Check sheet for the modelled part. Datum: model origin and axes. Units: mm. Coordinates: 2 decimals unless noted, no trailing zeros. Loops run counter-clockwise (first coordinate to the right, second up) from the corner with the lowest first, then second, coordinate; pieces in that order, holes last. Notation, with made-up numbers: (-14, -31) - (45, -31) arc R24 ccw to (45, -20) - close; hole circle Ø7 at (54, 57.25). An arc over 180 degrees is marked (long way). Use a Markdown table: item, result. Add a question column.
1) Sectioned sample at A-A, the plane y = 7.5. Enter the section's corners in (x, z).
2) Draft check along X on faces 1 (the flat face through (4, 13, 12.7)), 2 (the flat face through (10.2, 7.7, -10.2)), 3 (the cylindrical face through (-4.42, 11.56, -9.35)). Enter one of: pulls with the +X half, pulls with the -X half, needs draft (parallel to the pull), parting line crosses it, or undercut.
3) Sectioned sample at B-B, the plane z = 0. Enter the section's corners in (x, y), then the cut area to 3 significant figures.
4) Sectioned sample at D-D, the plane y = -1.75. Enter the section's corners in (x, z).
5) Sectioned sample at C-C, the plane x = -8.5. Enter the section's corners in (y, z).
6) Thickness scan on line 1 (Y direction, x = 0, z = -8); line 2 (Z direction, x = 0, y = 18). Record the ranges inside material, lowest first.
7) Go/stop test with flat-tipped pins: P1, Ø2, axis at y = 12.5, z = -9, coming from the +X side; P2, Ø11, axis at x = 0, z = 0, coming from the -Y side; P3, Ø3, axis at y = 3, z = -10, coming from the +X side. Record where each tip stops, or that it passes through.
from build123d import *

# Parameters (mm, degrees)
SKETCH1_R           = 6
BOSS_EXTRUDE1_DEPTH = 15
SKETCH2_R           = 6
CUT_EXTRUDE1_DEPTH  = 32
SKETCH3_R           = 6
CUT_EXTRUDE2_DEPTH  = 32
BOSS_EXTRUDE2_DEPTH = 5
BOSS_EXTRUDE3_DEPTH = 5
CUT_EXTRUDE3_START  = -31
SKETCH8_R           = 6
CUT_EXTRUDE3_DEPTH  = 31


with BuildPart() as part:
    # Sketch1 → Boss-Extrude1 (new body)
    with BuildSketch(Plane(origin=(0, 0, 0), x_dir=(1, 0, 0), z_dir=(0, 1, 0))):
        Polygon((-7.7, 12.7), (-12.7, 7.7), (-12.7, -7.7), (-7.7, -12.7), (7.7, -12.7), (12.7, -7.7), (12.7, 7.7), (7.7, 12.7), align=None)
        with Locations(Location((0, 0, 0), (0, 0, 270))):
            Circle(SKETCH1_R, mode=Mode.SUBTRACT)
    extrude(amount=BOSS_EXTRUDE1_DEPTH)

    # Sketch2 → Cut-Extrude1 (cut)
    with BuildSketch(Plane.XY.offset(12.7)):
        with Locations((0, 7.5)):
            Circle(SKETCH2_R)
    extrude(amount=-CUT_EXTRUDE1_DEPTH, mode=Mode.SUBTRACT)

    # Sketch3 → Cut-Extrude2 (cut)
    with BuildSketch(Plane.ZY.offset(12.7)):
        with Locations((0, 7.5)):
            Circle(SKETCH3_R)
    extrude(amount=-CUT_EXTRUDE2_DEPTH, mode=Mode.SUBTRACT)

    # Sketch6 → Boss-Extrude2 (add)
    with BuildSketch(Plane(origin=(0, 15, 0), x_dir=(1, 0, 0), z_dir=(0, 1, 0))):
        Polygon((7.7, 12.7), (-7.7, 12.7), (-12.7, 7.7), (-12.7, -7.7), (-7.7, -12.7), (7.7, -12.7), (12.7, -7.7), (12.7, 7.7), align=None)
    extrude(amount=BOSS_EXTRUDE2_DEPTH)

    # Sketch7 → Boss-Extrude3 (add)
    with BuildSketch(Plane.XZ):
        Polygon((-7.7, -12.7), (7.7, -12.7), (12.7, -7.7), (12.7, 7.7), (7.7, 12.7), (-7.7, 12.7), (-12.7, 7.7), (-12.7, -7.7), align=None)
    extrude(amount=BOSS_EXTRUDE3_DEPTH)

    # Sketch8 → Cut-Extrude3 (cut)
    with BuildSketch(Plane(origin=(0, 20, 0), x_dir=(1, 0, 0), z_dir=(0, 1, 0)).offset(CUT_EXTRUDE3_START)):
        with Locations(Location((0, 0, 0), (0, 0, 135))):
            Circle(SKETCH8_R)
    extrude(amount=CUT_EXTRUDE3_DEPTH, mode=Mode.SUBTRACT)


solid = part.part
Solved:
| question | item | result |
|---|---|---|
| 1 | outline | (-12.7, -7.7) - (-7.7, -12.7) - (-6, -12.7) - (-6, -6) - (-12.7, -6) - close; (-12.7, 6) - (-6, 6) - (-6, 12.7) - (-7.7, 12.7) - (-12.7, 7.7) - close; (6, -12.7) - (7.7, -12.7) - (12.7, -7.7) - (12.7, -6) - (6, -6) - close; (6, 6) - (12.7, 6) - (12.7, 7.7) - (7.7, 12.7) - (6, 12.7) - close |
| 2 | face 1 | needs draft |
| 2 | face 2 | pulls with the +X half |
| 2 | face 3 | undercut |
| 3 | outline | (-12.7, -5) - (-6, -5) - (-6, 1.5) - (-12.7, 1.5) - close; (-12.7, 13.5) - (-6, 13.5) - (-6, 20) - (-12.7, 20) - close; (6, -5) - (12.7, -5) - (12.7, 1.5) - (6, 1.5) - close; (6, 13.5) - (12.7, 13.5) - (12.7, 20) - (6, 20) - close |
| 3 | area | 174 mm2 |
| 4 | outline | (-12.7, -7.7) - (-7.7, -12.7) - (7.7, -12.7) - (12.7, -7.7) - (12.7, 7.7) - (7.7, 12.7) - (-7.7, 12.7) - (-12.7, 7.7) - close; hole circle Ø12 at (0, 0) |
| 5 | outline | (-5, -11.9) - (20, -11.9) - (20, 11.9) - (-5, 11.9) - close; hole circle Ø12 at (7.5, 0) |
| 6 | line 1 | y = -5 to 1.5, 13.5 to 20 |
| 6 | line 2 | z = -12.7 to -6, 6 to 12.7 |
| 7 | P1 | stops at x = 12.4 |
| 7 | P2 | passes through |
| 7 | P3 | stops at x = 11.9 |
